Input: part model. Units: mm. Frame: model coordinates. A direction names the side the tool comes from. Give positions to 0.01 mm unless a question says otherwise; leave off trailing zeros. Write each loop counter-clockwise with the first axis right and the second up, starting at its lowest first coordinate (ties: lowest second). Pieces come first, ordered by that corner, then holes. Notation, with made-up numbers: (41, -23.5) - (91, -23.5) arc R16 cw to (91, -17.5) - close; hole circle Ø1 at (-5, -39). An arc over 180 degrees is marked (long way). Use a Markdown table: item, result. Add a question column.
1. Section query C-C, the plane x = 183.5. Return loops of the section in (y, z).
2. Mould query, pull axis X, two halves, no side actions, for faces 1 (the flat face through (26, -57, 2)), 2 (the flat face through (110, -16, 33)), 3 (the flat face through (10, -16, 33)). Classes: released by +X, released by -X, zero draft, split by the parting line, or undercut.
3. Set-up query: faces 4 (the cylindrical face through (202.154, -10.947, 14.084)), 5 (the flat face through (112, -43, 10)), 6 (the flat face through (10, -80, 37)), 7 (the cylindrical face through (209, -82, 38)), 8 (the flat face through (59, -6, 33)). Return all of +Z, -Z, +X, -X, +Y, -Y with unobstructed straight access to the full face (end or side cutting, diameter ignored); none if empty.
4. Pin query (flat end, axial travel): pin 1 (8 mm diameter, centred on y = -14.5, z = 26.5, fed in from -X); pin 2 (1 mm diameter, centred on x = 77, z = 22.5, fed in from -Y); pin 3 (19.5 mm diameter, centred on x = 195, y = -81, fed in from +Z); pin 4 (16 mm diameter, centred on x = 46, y = -17, fed in from +Z). Return the tip coordinate at first contact, or that it passes through.
5. Section query B-B, the plane x = 137. Return loops of the section in (y, z), plus the area to 3 significant figures.
6. Section query D-D, the plane x = 82.5. Return loops of the section in (y, z), plus the area to 3 significant figures.
7. Section query A-A, the plane z = 32. Return loops of the section in (x, y), plus the area to 3 significant figures.
8. Material intervals for probe 1 along Y at (x, z) = (195, 4); probe 2 along Y at (x, z) = (19.5, 29); probe 3 along Y at (x, z) = (131, 16.5), sorted ascending.
```python
from build123d import *

# Parameters (mm, degrees)
SKETCH1_W           = 210
SKETCH1_H           = 90
BOSS_EXTRUDE1_DEPTH = 20
SKETCH2_R           = 1.6
CUT_EXTRUDE1_DEPTH  = 20
SKETCH3_W           = 110
SKETCH3_H           = 10
BOSS_EXTRUDE2_DEPTH = 30
SKETCH4_W           = 100
SKETCH4_H           = 20
BOSS_EXTRUDE3_DEPTH = 26
SKETCH5_R           = 2.25
CUT_EXTRUDE2_DEPTH  = 234.057932712
SKETCH7_W           = 80
SKETCH7_H           = 64
CUT_EXTRUDE3_DEPTH  = 16
SKETCH8_R           = 7.5
CUT_EXTRUDE4_DEPTH  = 12
SKETCH9_R           = 7.5
CUT_EXTRUDE5_DEPTH  = 42
SKETCH10_W          = 68
SKETCH10_H          = 45
CUT_EXTRUDE6_DEPTH  = 46
SKETCH11_W          = 20
SKETCH11_H          = 10
BOSS_EXTRUDE5_DEPTH = 30
FILLET1_R           = 10
SKETCH12_W          = 68
SKETCH12_H          = 46
CUT_EXTRUDE7_DEPTH  = 30
FILLET2_R           = 5
FILLET3_R           = 5
FILLET4_R           = 3
FILLET5_R           = 3


with BuildPart() as part:
    # Sketch1 → Boss-Extrude1 (new body)
    with BuildSketch(Plane.XY):
        with Locations((105, -45)):
            Rectangle(SKETCH1_W, SKETCH1_H)
    extrude(amount=BOSS_EXTRUDE1_DEPTH)

    # Sketch2 → Cut-Extrude1 (cut)
    with BuildSketch(Plane.XY.offset(20)):
        with Locations((195, -13.2)):
            Circle(SKETCH2_R)
        with Locations((195, -81)):
            Circle(SKETCH2_R)
    extrude(amount=-CUT_EXTRUDE1_DEPTH, mode=Mode.SUBTRACT)

    # Sketch3 → Boss-Extrude2 (add)
    with BuildSketch(Plane.XY.offset(20)):
        with Locations((155, -85)):
            Rectangle(SKETCH3_W, SKETCH3_H)
    extrude(amount=BOSS_EXTRUDE2_DEPTH)

    # Sketch4 → Boss-Extrude3 (add)
    with BuildSketch(Plane.XY.offset(20)):
        with Locations((60, -16)):
            Rectangle(SKETCH4_W, SKETCH4_H)
    extrude(amount=BOSS_EXTRUDE3_DEPTH)

    # Sketch5 → Cut-Extrude2 (cut, through all)
    with BuildSketch(Plane.XY.offset(46)):
        with Locations((100.5, -16)):
            Circle(SKETCH5_R)
        with Locations((19.5, -16)):
            Circle(SKETCH5_R)
    extrude(amount=-CUT_EXTRUDE2_DEPTH, mode=Mode.SUBTRACT)

    # Sketch7 → Cut-Extrude3 (cut)
    with BuildSketch(Plane.XY.offset(20)):
        with Locations((60, -58)):
            Rectangle(SKETCH7_W, SKETCH7_H)
    extrude(amount=-CUT_EXTRUDE3_DEPTH, mode=Mode.SUBTRACT)

    # Sketch8 → Cut-Extrude4 (cut)
    with BuildSketch(Plane.XY.offset(20)):
        with Locations((195, -13.2)):
            Circle(SKETCH8_R)
    extrude(amount=-CUT_EXTRUDE4_DEPTH, mode=Mode.SUBTRACT)

    # Sketch9 → Cut-Extrude5 (cut)
    with BuildSketch(Plane.XY.offset(50)):
        with Locations((195, -81)):
            Circle(SKETCH9_R)
    extrude(amount=-CUT_EXTRUDE5_DEPTH, mode=Mode.SUBTRACT)

    # Sketch10 → Cut-Extrude6 (cut)
    with BuildSketch(Plane.XY.offset(20)):
        with Locations((146, -42.5)):
            Rectangle(SKETCH10_W, SKETCH10_H)
    extrude(amount=-CUT_EXTRUDE6_DEPTH, mode=Mode.SUBTRACT)

    # Sketch11 → Boss-Extrude5 (add)
    with BuildSketch(Plane.XY.offset(20)):
        with Locations((10, -85)):
            Rectangle(SKETCH11_W, SKETCH11_H)
    extrude(amount=BOSS_EXTRUDE5_DEPTH)

    # Fillet1
    fillet1_edges = [part.edges().sort_by_distance(p)[0] for p in [
        (0, 0, 10),
        (210, 0, 10),
    ]]
    fillet(fillet1_edges, radius=FILLET1_R)

    # Sketch12 → Cut-Extrude7 (cut)
    with BuildSketch(Plane.XY.offset(4)):
        with Locations((60, -57)):
            Rectangle(SKETCH12_W, SKETCH12_H)
    extrude(amount=-CUT_EXTRUDE7_DEPTH, mode=Mode.SUBTRACT)

    # Fillet2
    fillet2_edges = [part.edges().sort_by_distance(p)[0] for p in [
        (0, -80, 35),
        (20, -80, 35),
        (210, -80, 35),
        (100, -80, 35),
    ]]
    fillet(fillet2_edges, radius=FILLET2_R)

    # Fillet3
    # the kernel refuses this fillet: 5 mm, written as the material it adds along each edge
    with BuildSketch(Plane(origin=(189.933034374, -80, 20), x_dir=(0, 1, 0), z_dir=(1, 0, 0))) as fillet3_piece_1_section:
        with BuildLine():
            CenterArc((FILLET3_R, FILLET3_R), FILLET3_R, 180, 90)
            Line((0, FILLET3_R), (0, 0))
            Line((0, 0), (FILLET3_R, 0))
        make_face()
    fillet3_piece_1 = extrude(amount=15.066965626, mode=Mode.PRIVATE)
    fillet3_piece_1 = fillet3_piece_1 - Plane(origin=(195, -81, 20.004383527), x_dir=(1, 0, 0), z_dir=(0, 0, 1)) * Cylinder(7.5, 51, mode=Mode.PRIVATE)
    add(fillet3_piece_1)
    with BuildSketch(Plane(origin=(15, -80, 20), x_dir=(0, 1, 0), z_dir=(-1, 0, 0))) as fillet3_piece_2:
        with BuildLine():
            CenterArc((FILLET3_R, -FILLET3_R), FILLET3_R, 90, 90)
            Line((0, -FILLET3_R), (0, 0))
            Line((0, 0), (FILLET3_R, 0))
        make_face()
    extrude(amount=10)
    with BuildSketch(Plane(origin=(205, -85, 20), x_dir=(-0.801744239297649, -0.5976672776328267, 0), z_dir=(-0.5976672776328267, 0.801744239297649, 0))) as fillet3_piece_3_section:
        with BuildLine():
            CenterArc((5 + FILLET3_R, FILLET3_R), FILLET3_R, 180, 90)
            Line((5, FILLET3_R), (5, 0))
            Line((5, 0), (5 + FILLET3_R, 0))
        make_face()
    fillet3_piece_3 = revolve(axis=Axis((205, -85, 20), (0, 0, 1)), revolution_arc=233.296989237, mode=Mode.PRIVATE)
    fillet3_piece_3 = split(fillet3_piece_3, bisect_by=Plane(origin=(208.749694825, -90, 21.558141558), z_dir=(0, 1, 0)), keep=Keep.TOP, mode=Mode.PRIVATE)
    fillet3_piece_3 = split(fillet3_piece_3, bisect_by=Plane(origin=(210, -81.250305307, 21.558141558), z_dir=(-1, 0, 0)), keep=Keep.TOP, mode=Mode.PRIVATE)
    add(fillet3_piece_3)
    with BuildSketch(Plane(origin=(105, -85, 20), x_dir=(0, 1, 0), z_dir=(1, 0, 0))) as fillet3_piece_4_section:
        with BuildLine():
            CenterArc((5 + FILLET3_R, FILLET3_R), FILLET3_R, 180, 90)
            Line((5, FILLET3_R), (5, 0))
            Line((5, 0), (5 + FILLET3_R, 0))
        make_face()
    fillet3_piece_4 = revolve(axis=Axis((105, -85, 20), (0, 0, 1)), revolution_arc=233.296989237, mode=Mode.PRIVATE)
    fillet3_piece_4 = split(fillet3_piece_4, bisect_by=Plane(origin=(103.049091377, -90, 20.836500951), z_dir=(0, 1, 0)), keep=Keep.TOP, mode=Mode.PRIVATE)
    fillet3_piece_4 = split(fillet3_piece_4, bisect_by=Plane(origin=(100, -78.901123736, 20.836500951), z_dir=(1, 0, 0)), keep=Keep.TOP, mode=Mode.PRIVATE)
    add(fillet3_piece_4)
    with BuildSketch(Plane(origin=(15, -85, 20), x_dir=(0, 1, 0), z_dir=(-1, 0, 0))) as fillet3_piece_5_section:
        with BuildLine():
            CenterArc((5 + FILLET3_R, -FILLET3_R), FILLET3_R, 90, 90)
            Line((5, -FILLET3_R), (5, 0))
            Line((5, 0), (5 + FILLET3_R, 0))
        make_face()
    fillet3_piece_5 = revolve(axis=Axis((15, -85, 20), (0, 0, -1)), revolution_arc=233.296989237, mode=Mode.PRIVATE)
    fillet3_piece_5 = split(fillet3_piece_5, bisect_by=Plane(origin=(16.950908623, -90, 20.836500951), z_dir=(0, 1, 0)), keep=Keep.TOP, mode=Mode.PRIVATE)
    fillet3_piece_5 = split(fillet3_piece_5, bisect_by=Plane(origin=(20, -78.901123736, 20.836500951), z_dir=(-1, 0, 0)), keep=Keep.TOP, mode=Mode.PRIVATE)
    add(fillet3_piece_5)
    with BuildSketch(Plane(origin=(5, -85, 20), x_dir=(0.8017442392976476, -0.5976672776328283, 0), z_dir=(0.5976672776328283, 0.8017442392976476, 0))) as fillet3_piece_6_section:
        with BuildLine():
            CenterArc((5 + FILLET3_R, -FILLET3_R), FILLET3_R, 90, 90)
            Line((5, -FILLET3_R), (5, 0))
            Line((5, 0), (5 + FILLET3_R, 0))
        make_face()
    fillet3_piece_6 = revolve(axis=Axis((5, -85, 20), (0, 0, -1)), revolution_arc=233.296989237, mode=Mode.PRIVATE)
    fillet3_piece_6 = split(fillet3_piece_6, bisect_by=Plane(origin=(1.250305308, -90, 21.55814164), z_dir=(0, 1, 0)), keep=Keep.TOP, mode=Mode.PRIVATE)
    fillet3_piece_6 = split(fillet3_piece_6, bisect_by=Plane(origin=(0, -81.250305308, 21.55814164), z_dir=(1, 0, 0)), keep=Keep.TOP, mode=Mode.PRIVATE)
    add(fillet3_piece_6)
    with BuildSketch(Plane(origin=(105, -80, 20), x_dir=(0, 1, 0), z_dir=(1, 0, 0))) as fillet3_piece_7_section:
        with BuildLine():
            CenterArc((FILLET3_R, FILLET3_R), FILLET3_R, 180, 90)
            Line((0, FILLET3_R), (0, 0))
            Line((0, 0), (FILLET3_R, 0))
        make_face()
    fillet3_piece_7 = extrude(amount=95.066965626, mode=Mode.PRIVATE)
    fillet3_piece_7 = fillet3_piece_7 - Plane(origin=(195, -81, 21.114667371), x_dir=(1, 0, 0), z_dir=(0, 0, 1)) * Cylinder(7.5, 211, mode=Mode.PRIVATE)
    add(fillet3_piece_7)

    # Fillet4
    fillet4_edges = [part.edges().sort_by_distance(p)[0] for p in [
        (180, -20, 10),
        (180, -65, 10),
        (26, -80, 2),
        (26, -34, 2),
        (94, -34, 2),
        (94, -80, 2),
        (20, -26, 12),
        (100, -26, 12),
        (112, -65, 10),
        (112, -20, 10),
    ]]
    fillet(fillet4_edges, radius=FILLET4_R)

    # Fillet5
    fillet5_edges = [part.edges().sort_by_distance(p)[0] for p in [
        (10, -6, 33),
        (10, -26, 33),
        (110, -26, 33),
        (110, -6, 33),
    ]]
    fillet(fillet5_edges, radius=FILLET5_R)


solid = part.part
```
Result sheet:
| question | item | result |
|---|---|---|
| 1 | outline | (-90, 0) - (0, 0) - (0, 20) - (-75, 20) arc R5 cw to (-80, 25) - (-80, 50) - (-90, 50) - close |
| 2 | face 1 | undercut |
| 2 | face 2 | released by +X |
| 2 | face 3 | released by -X |
| 3 | face 4 | +Z |
| 3 | face 5 | +Z, -Z |
| 3 | face 6 | +Z, +X, -X |
| 3 | face 7 | +Z, +X, +Y |
| 3 | face 8 | +Z, +X, -X, +Y |
| 4 | pin 1 | stops at x = 10 |
| 4 | pin 2 | stops at y = -26 |
| 4 | pin 3 | stops at z = 50 |
| 4 | pin 4 | stops at z = 46 |
| 5 | outline | (-90, 0) - (-65, 0) - (-65, 20) - (-75, 20) arc R5 cw to (-80, 25) - (-80, 50) - (-90, 50) - close; (-20, 0) - (0, 0) - (0, 20) - (-20, 20) - close |
| 5 | area | 1,210 mm² |
| 6 | outline | (-90, 0) - (-80, 0) - (-80, 4) - (-90, 4) - close; (-34, 0) - (0, 0) - (0, 20) - (-6, 20) - (-6, 46) - (-26, 46) - (-26, 4) - (-34, 4) - close |
| 6 | area | 1,110 mm² |
| 7 | outline | (0, -90) - (20, -90) - (20, -85) arc R5 ccw to (15, -80) - (5, -80) arc R5 ccw to (0, -85) - close; (10, -23) arc R3 ccw to (13, -26) - (107, -26) arc R3 ccw to (110, -23) - (110, -9) arc R3 ccw to (107, -6) - (13, -6) arc R3 ccw to (10, -9) - close; (100, -90) - (210, -90) - (210, -85) arc R5 ccw to (205, -80) - (202.43, -80) arc R7.5 cw (long way) to (187.57, -80) - (105, -80) arc R5 ccw to (100, -85) - close; hole circle Ø4.5 at (19.5, -16); hole circle Ø4.5 at (100.5, -16) |
| 7 | area | 3,140 mm² |
| 8 | probe 1 | y = -90 to -82.6, -79.4 to -14.8, -11.6 to 0 |
| 8 | probe 2 | y = -90 to -82.82, -26 to -18.25, -13.75 to -6 |
| 8 | probe 3 | y = -90 to -65, -20 to 0 |
